```python
from build123d import *

# Parameters (mm, degrees)
SKETCH1_W               = 1030
SKETCH1_H               = 1035
BOSS_EXTRUDE1_DEPTH     = 72
SKETCH2_R               = 7.5
BOSS_EXTRUDE2_DEPTH     = 30
SKETCH3_W               = 24
SKETCH3_H               = 101
BOSS_EXTRUDE3_DEPTH     = 12
SKETCH4_W               = 24
SKETCH4_H               = 12
BOSS_EXTRUDE4_DEPTH     = 100
LPATTERN1_COUNT         = 2
LPATTERN1_PITCH         = 600
MIRROR2_COPY_1_SKETCH_W = 24
MIRROR2_COPY_1_SKETCH_H = 101
MIRROR2_COPY_1_DEPTH    = 12
MIRROR2_COPY_2_SKETCH_W = 24
MIRROR2_COPY_2_SKETCH_H = 12
MIRROR2_COPY_2_DEPTH    = 100
SKETCH6_R               = 7.5
BOSS_EXTRUDE5_DEPTH     = 30
LPATTERN2_COUNT         = 10
LPATTERN2_PITCH         = 93.6364
MIRROR3_COPY_1_SKETCH_R = 7.5
MIRROR3_COPY_1_DEPTH    = 30
MIRROR3_COPY_2_SKETCH_R = 7.5
MIRROR3_COPY_2_DEPTH    = 30
MIRROR3_COPY_3_SKETCH_R = 7.5
MIRROR3_COPY_3_DEPTH    = 30
MIRROR3_COPY_4_SKETCH_R = 7.5
MIRROR3_COPY_4_DEPTH    = 30
MIRROR3_COPY_5_SKETCH_R = 7.5
MIRROR3_COPY_5_DEPTH    = 30
MIRROR3_COPY_6_SKETCH_R = 7.5
MIRROR3_COPY_6_DEPTH    = 30
MIRROR3_COPY_7_SKETCH_R = 7.5
MIRROR3_COPY_7_DEPTH    = 30
MIRROR3_COPY_8_SKETCH_R = 7.5
MIRROR3_COPY_8_DEPTH    = 30
MIRROR3_COPY_9_SKETCH_R = 7.5
MIRROR3_COPY_9_DEPTH    = 30


with BuildPart() as part:
    # Sketch1 → Boss-Extrude1 (new body)
    with BuildSketch(Plane.XY):
        Rectangle(SKETCH1_W, SKETCH1_H)
    extrude(amount=BOSS_EXTRUDE1_DEPTH)

    # Sketch2 → Boss-Extrude2 (add)
    with BuildSketch(Plane(origin=(515, 0, 0), x_dir=(0, 0, -1), z_dir=(1, 0, 0))):
        with Locations(Location((-36, 378.5, 0), (0, 0, 180))):
            Circle(SKETCH2_R)
    boss_extrude2 = extrude(amount=BOSS_EXTRUDE2_DEPTH)

    # Sketch3 → Boss-Extrude3 (add)
    with BuildSketch(Plane(origin=(515, 0, 0), x_dir=(0, 0, -1), z_dir=(1, 0, 0))):
        with Locations((-36, 233)):
            Rectangle(SKETCH3_W, SKETCH3_H)
    boss_extrude3 = extrude(amount=BOSS_EXTRUDE3_DEPTH)

    # Sketch4 → Boss-Extrude4 (add)
    with BuildSketch(Plane(origin=(527, 0, 0), x_dir=(0, 0, -1), z_dir=(1, 0, 0))):
        with Locations((-36, 188.5)):
            Rectangle(SKETCH4_W, SKETCH4_H)
    boss_extrude4 = extrude(amount=BOSS_EXTRUDE4_DEPTH)

    # LPattern1: Boss-Extrude3, Boss-Extrude4 ×2
    with Locations(*[(0, -i * LPATTERN1_PITCH, 0) for i in range(1, LPATTERN1_COUNT)]):
        add(boss_extrude3)
        add(boss_extrude4)

    # Mirror2: Boss-Extrude2, Boss-Extrude3, Boss-Extrude4 across plane
    add(boss_extrude2.mirror(Plane(origin=(0, 0, 0), x_dir=(0, 0, 1), z_dir=(1, 0, 0))))
    add(boss_extrude3.mirror(Plane(origin=(0, 0, 0), x_dir=(0, 0, 1), z_dir=(1, 0, 0))))
    add(boss_extrude4.mirror(Plane(origin=(0, 0, 0), x_dir=(0, 0, 1), z_dir=(1, 0, 0))))

    # Mirror2 copy 1 sketch → Mirror2 copy 1 (add)
    with BuildSketch(Plane(origin=(-515, -600, 0), x_dir=(0, 0, -1), z_dir=(-1, 0, 0))):
        with Locations((-36, -233)):
            Rectangle(MIRROR2_COPY_1_SKETCH_W, MIRROR2_COPY_1_SKETCH_H)
    extrude(amount=MIRROR2_COPY_1_DEPTH)

    # Mirror2 copy 2 sketch → Mirror2 copy 2 (add)
    with BuildSketch(Plane(origin=(-527, -600, 0), x_dir=(0, 0, -1), z_dir=(-1, 0, 0))):
        with Locations((-36, -188.5)):
            Rectangle(MIRROR2_COPY_2_SKETCH_W, MIRROR2_COPY_2_SKETCH_H)
    extrude(amount=MIRROR2_COPY_2_DEPTH)

    # Sketch6 → Boss-Extrude5 (add)
    with BuildSketch(Plane(origin=(0, 517.5, 0), x_dir=(1, 0, 0), z_dir=(0, 1, 0))):
        with Locations(Location((421.3636, -36, 0), (0, 0, 90))):
            Circle(SKETCH6_R)
    boss_extrude5 = extrude(amount=BOSS_EXTRUDE5_DEPTH)

    # LPattern2: Boss-Extrude5 ×10
    with Locations(*[(-i * LPATTERN2_PITCH, 0, 0) for i in range(1, LPATTERN2_COUNT)]):
        add(boss_extrude5)

    # Mirror3: Boss-Extrude5 across plane
    add(boss_extrude5.mirror(Plane.ZX))

    # Mirror3 copy 1 sketch → Mirror3 copy 1 (add)
    with BuildSketch(Plane(origin=(-93.6364, -517.5, 0), x_dir=(1, 0, 0), z_dir=(0, -1, 0))):
        with Locations((421.3636, 36)):
            Circle(MIRROR3_COPY_1_SKETCH_R)
    extrude(amount=MIRROR3_COPY_1_DEPTH)

    # Mirror3 copy 2 sketch → Mirror3 copy 2 (add)
    with BuildSketch(Plane(origin=(-187.2728, -517.5, 0), x_dir=(1, 0, 0), z_dir=(0, -1, 0))):
        with Locations((421.3636, 36)):
            Circle(MIRROR3_COPY_2_SKETCH_R)
    extrude(amount=MIRROR3_COPY_2_DEPTH)

    # Mirror3 copy 3 sketch → Mirror3 copy 3 (add)
    with BuildSketch(Plane(origin=(-280.9092, -517.5, 0), x_dir=(1, 0, 0), z_dir=(0, -1, 0))):
        with Locations((421.3636, 36)):
            Circle(MIRROR3_COPY_3_SKETCH_R)
    extrude(amount=MIRROR3_COPY_3_DEPTH)

    # Mirror3 copy 4 sketch → Mirror3 copy 4 (add)
    with BuildSketch(Plane(origin=(-374.5456, -517.5, 0), x_dir=(1, 0, 0), z_dir=(0, -1, 0))):
        with Locations((421.3636, 36)):
            Circle(MIRROR3_COPY_4_SKETCH_R)
    extrude(amount=MIRROR3_COPY_4_DEPTH)

    # Mirror3 copy 5 sketch → Mirror3 copy 5 (add)
    with BuildSketch(Plane(origin=(-468.182, -517.5, 0), x_dir=(1, 0, 0), z_dir=(0, -1, 0))):
        with Locations((421.3636, 36)):
            Circle(MIRROR3_COPY_5_SKETCH_R)
    extrude(amount=MIRROR3_COPY_5_DEPTH)

    # Mirror3 copy 6 sketch → Mirror3 copy 6 (add)
    with BuildSketch(Plane(origin=(-561.8184, -517.5, 0), x_dir=(1, 0, 0), z_dir=(0, -1, 0))):
        with Locations((421.3636, 36)):
            Circle(MIRROR3_COPY_6_SKETCH_R)
    extrude(amount=MIRROR3_COPY_6_DEPTH)

    # Mirror3 copy 7 sketch → Mirror3 copy 7 (add)
    with BuildSketch(Plane(origin=(-655.4548, -517.5, 0), x_dir=(1, 0, 0), z_dir=(0, -1, 0))):
        with Locations((421.3636, 36)):
            Circle(MIRROR3_COPY_7_SKETCH_R)
    extrude(amount=MIRROR3_COPY_7_DEPTH)

    # Mirror3 copy 8 sketch → Mirror3 copy 8 (add)
    with BuildSketch(Plane(origin=(-749.0912, -517.5, 0), x_dir=(1, 0, 0), z_dir=(0, -1, 0))):
        with Locations((421.3636, 36)):
            Circle(MIRROR3_COPY_8_SKETCH_R)
    extrude(amount=MIRROR3_COPY_8_DEPTH)

    # Mirror3 copy 9 sketch → Mirror3 copy 9 (add)
    with BuildSketch(Plane(origin=(-842.7276, -517.5, 0), x_dir=(1, 0, 0), z_dir=(0, -1, 0))):
        with Locations((421.3636, 36)):
            Circle(MIRROR3_COPY_9_SKETCH_R)
    extrude(amount=MIRROR3_COPY_9_DEPTH)


solid = part.part
```
CAD build for the part. Positions are in the model's coordinates, mm. A direction names the side the tool comes from. Round coordinates to 2 decimals unless told otherwise and drop trailing zeros. Order: outer loops, then holes, each group sorted by start corner. A loop starts at its lowest first (then second) coordinate and runs counter-clockwise, first axis right, second up. Notation, with made-up numbers: (-3.5, 63) - (13.5, 63) arc R19 ccw to (13.5, 84) - close; hole circle Ø3 at (-26, 49.25). An arc over 180 degrees is marked (long way). Use CSV: the item, a comma, the result in double quotes. Start each with the question number.
1) Saw through at B-B (x = -484). List the corners of the cut face in (y, z).
2) Two-plate mould, pull along X, no slides. Class faces 1 (the flat face through (-546, 192, 24)), 2 (the flat face through (-7, -517.5, 35)): pulls with the +X half, pulls with the -X half, needs draft (parallel to the pull), parting line crosses it, or undercut.
3) Pin check, flat tips, straight feed: pin 1 Ø12 at (y, z) = (240.5, 35) entering from +X; pin 2 Ø4 at (y, z) = (-404.5, 48.5) entering from -X; pin 3 Ø21.5 at (y, z) = (-1, 40.5) entering from +X; pin 4 Ø5 at (y, z) = (-34, 46.5) entering from -X. Stop position of each tip, or through.
4) Wall check: L1, parallel to X at y = 81.5, z = 14; L2, parallel to Y at x = -340, z = 52.5; L3, parallel to X at y = -382, z = 43.5. Give the ranges that are in metal, low to high. Write a range as [from, to].
5) Tool access for faces 3 (the flat face through (546, -408, 48)), 4 (the flat face through (-550, -408, 48)), 5 (the flat face through (-550, -408, 24)), 6 (the flat face through (546, -408, 24)): list every direction of +Z, -Z, +X, -X, +Y, -Y with a clear straight run to the whole face (end or side of a thin tool).
6) Saw through at A-A (y = -287.5). List the corners of the cut face in (x, z), and give its area (3 significant figures).
Values follow:
1,outline,"(-517.5, 0) - (517.5, 0) - (517.5, 72) - (-517.5, 72) - close"
2,face 1,"needs draft"
2,face 2,"undercut"
3,pin 1,"stops at x = 527"
3,pin 2,"stops at x = -627"
3,pin 3,"stops at x = 515"
3,pin 4,"stops at x = -515"
4,L1,"x = [-515, 515]"
4,L2,"y = [-517.5, 517.5]"
4,L3,"x = [-527, 527]"
5,face 3,"+Z, +X, +Y, -Y"
5,face 4,"+Z, -X, +Y, -Y"
5,face 5,"-Z, -X, +Y, -Y"
5,face 6,"-Z, +X, +Y, -Y"
6,outline,"(-515, 0) - (515, 0) - (515, 72) - (-515, 72) - close"
6,area,"74,200 mm2"
